Can you work these out from the model? Positions are in its coordinate system, mm. A direction names the side the tool comes from. Give positions to 0.01 mm unless a question says otherwise; leave off trailing zeros. Order: outer loops, then holes, each group sorted by start corner. A loop starts at its lowest first (then second) coordinate and runs counter-clockwise, first axis right, second up. Notation, with made-up numbers: (50, 68) - (54, 68) arc R27 ccw to (54, 97) - close; hole circle Ø7 at (74.25, -18). An arc over 180 degrees is marked (long way). Answer as a JSON object with one key per item and string values.
Autodesk Inventor part; units mm, degrees
ref_plane "YZ Plane" through (0, 0, 0) normal (1, 0, 0) x (0, 1, 0)
ref_plane "XZ Plane" through (0, 0, 0) normal (0, 1, 0) x (-1, 0, 0)
ref_plane "XY Plane" through (0, 0, 0) normal (0, 0, 1) x (1, 0, 0)
sketch "Sketch1" plane through (0, 0, 0) normal (0, 1, 0) x (-1, 0, 0)
  circle A0 centre (0, 0) radius 80
  dimension "d0" = 160
extrude "Extrusion1" add sketch "Sketch1" along normal blind 4
sketch "Sketch2" plane through (0, 0, 0) normal (0, -1, 0) x (1, 0, 0)
  point P0 (0, 0)
sketch "Sketch4" plane through (0, 0, 0) normal (0, -1, 0) x (1, 0, 0)
  circle A0 centre (0, 0) radius 5.5
  dimension "d7" = 11
extrude "Extrusion3" add sketch "Sketch4" along normal blind 5
sketch "Sketch5" plane through (0, 0, 0) normal (0, -1, 0) x (1, 0, 0)
  point P0 (0, 0)
sketch "Sketch8" plane through (0, -5, 0) normal (0, -1, 0) x (1, 0, 0)
  line L0 (3.9692, 4.8706) -> (31.1403, 4.8706)
  line L1 (31.1403, 4.8706) -> (31.1403, -5.1294)
  line L2 (31.1403, -5.1294) -> (3.9692, -5.1294)
  line L3 (3.9692, -5.1294) -> (3.9692, 4.8706)
  point P0 (0, 0)
  dimension "d15" = 10
extrude "Extrusion5" cut sketch "Sketch8" against normal blind 1
equation "\"d0\" = diamteru"
equation "\"d1\" = grosime"
equation "\"diamteru\" = 160"
equation "\"grosime\" = 4"
properties part number "pat" material "PET Plastic"
Q1. If we section it at B-B, the plane x = 0: Please give me the cut outline in (y, z).
Recorded:
{"outline": "(-5, -5.5) - (0, -5.5) - (0, -80) - (4, -80) - (4, 80) - (0, 80) - (0, 5.5) - (-5, 5.5) - close"}
Q2. If we section it at D-D, the plane z = 51: Please give me the cut outline in (x, y), then the cut area to 3 significant figures.
Recorded:
{"outline": "(-61.64, 0) - (61.64, 0) - (61.64, 4) - (-61.64, 4) - close", "area": "493 mm^2"}
Q3. Which directions (+Z, -Z, +X, -X, +Y, -Y) give clear straight access to the entire face, cutting with the end or side of a thin tool? Please do faces 1 (the face through (-5.495, -2.465, -0.242)), 2 (the face through (-1, -5, 0)).
Recorded:
{"face 1": "-Y", "face 2": "+Z, -Z, +X, -X, -Y"}
Q4. I need wall thicknesses on L1, parallel to Y at x = 48.5, z = -21; L2, parallel to X at y = 2.5, z = 46; L3, parallel to Z at x = -10, y = 2.25. Which ranges of each line are inside material? Lowest first, please.
Recorded:
{"L1": "y = 0 to 4", "L2": "x = -65.45 to 65.45", "L3": "z = -79.37 to 79.37"}
Q5. I'm going to push flat-ended pins straight in: pin 1 Ø12 at (x, z) = (-37, -41.5) entering from -Y; pin 2 Ø1.5 at (y, z) = (1.5, 38) entering from -X; pin 3 Ø0.8 at (x, z) = (5, -1.5) entering from -Y. Where does each tip first touch, or does it pass through?
Recorded:
{"pin 1": "stops at y = 0", "pin 2": "stops at x = -70.8", "pin 3": "stops at y = -4"}
Q6. If we section it at A-A, the plane z = 0: Please give me the cut outline in (x, y), then the cut area to 3 significant figures.
Recorded:
{"outline": "(-80, 0) - (-5.5, 0) - (-5.5, -5) - (3.97, -5) - (3.97, -4) - (5.5, -4) - (5.5, 0) - (80, 0) - (80, 4) - (-80, 4) - close", "area": "693 mm^2"}
Q7. If we section it at C-C, the plane y = 2.5: Please give me the cut outline in (x, z).
Recorded:
{"outline": "circle Ø160 at (0, 0)"}
